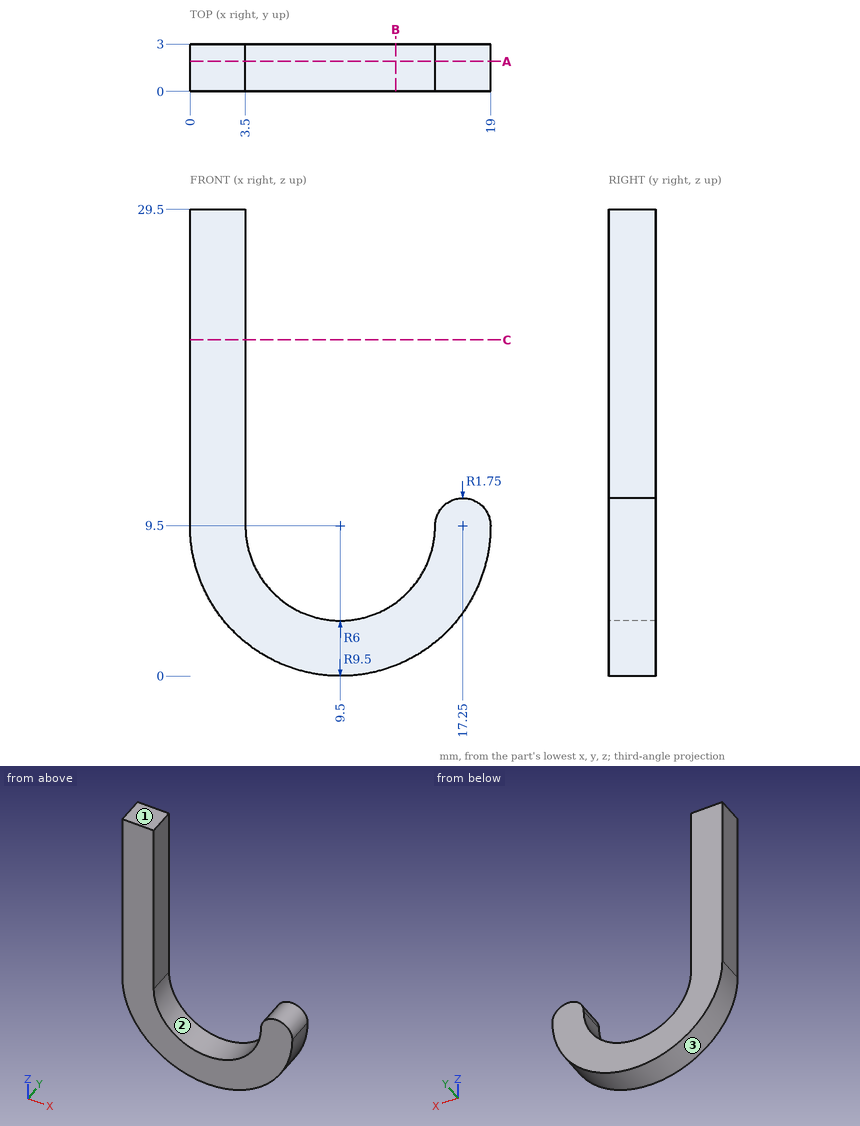
Design review of the part shown in the three views and the two pictorial views. Dimensions are in mm from the part's minimum x, y and z. Round coordinates to 2 decimals unless told otherwise and drop trailing zeros. Loops run counter-clockwise (first coordinate to the right, second up) from the corner with the lowest first, then second, coordinate; pieces in that order, holes last. Notation, with made-up numbers: (68.25, -24) -> (125.25, -24) arc R20 ccw to (125.25, 6) -> close; hole circle Ø5 at (-17.75, 60.5). An arc over 180 degrees is marked (long way). Return JSON: item names as keys, results as strings.
(1) Add section C-C on z = 21.25. Write out the cut boundary in (x, y), plus the area to 3 significant figures.
Solved:
{"outline": "(0, 0) -> (3.5, 0) -> (3.5, 3) -> (0, 3) -> close", "area": "10.5 mm2"}
(2) The part is to be moulded in two halves that separate along X. For the marked faces 1, 2 and 3, say which applies: released by +X, released by -X, zero draft, split by the parting line, or undercut.
Solved:
{"face 1": "zero draft", "face 2": "undercut", "face 3": "split by the parting line"}
(3) For pin 1 (1.5 mm diameter, centred on y = 1.5, z = 20, fed in from +X), flat-tipped, find the tip position at first contact; note if it passes through.
Solved:
{"pin 1": "x = 3.5"}
(4) Add section A-A on y = 1.9. Write out the cut boundary in (x, z).
Solved:
{"outline": "(0, 9.5) arc R9.5 ccw to (19, 9.5) arc R1.75 ccw to (15.5, 9.5) arc R6 cw to (3.5, 9.5) -> (3.5, 29.5) -> (0, 29.5) -> close"}
(5) Add section B-B on x = 13. Write out the cut boundary in (y, z), plus the area to 3 significant figures.
Solved:
{"outline": "(0, 0.67) -> (3, 0.67) -> (3, 4.63) -> (0, 4.63) -> close", "area": "11.9 mm2"}
(6) For line 1 (X direction, y = 1.2, z = 24); line 2 (X direction, y = 0.6, z = 4.25); line 3 (Z direction, x = 11, y = 0.65), list the stretches that pass through material, from the lowest coordinate up.
Solved:
{"line 1": "0 to 3.5", "line 2": "1.58 to 6.6, 12.4 to 17.42", "line 3": "0.12 to 3.69"}
